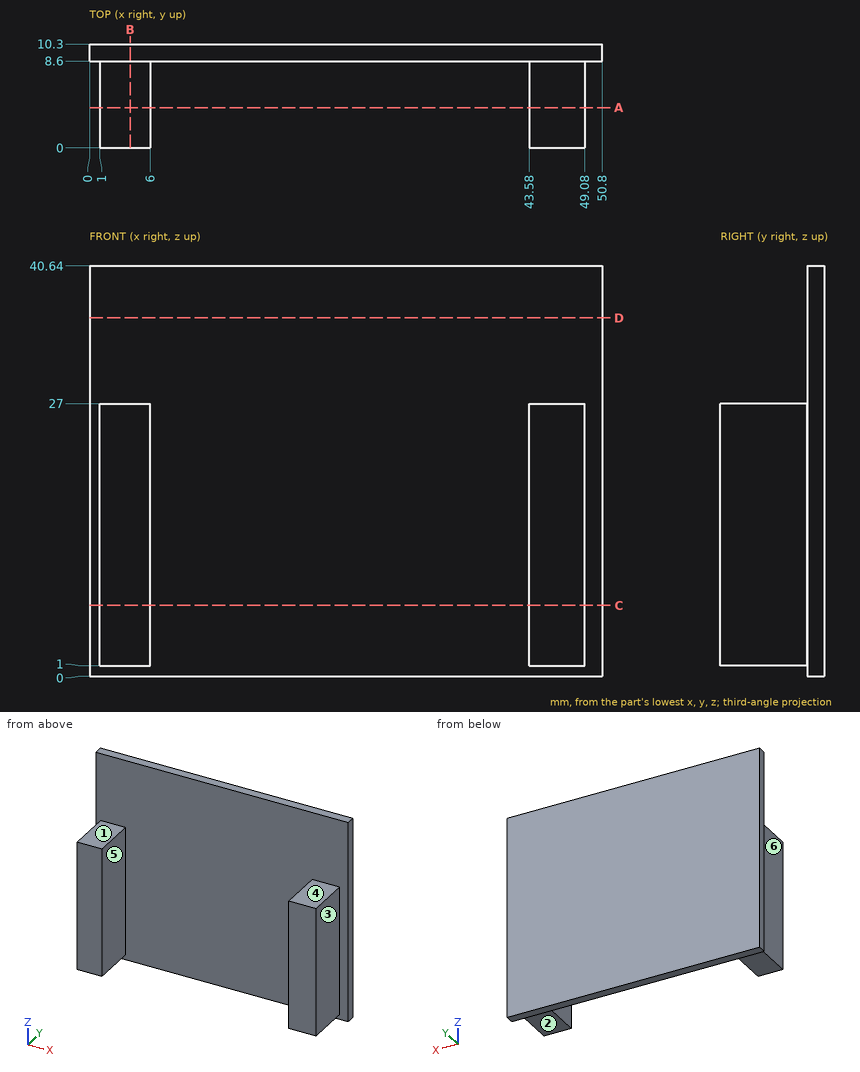
Design review of the part shown in the three views and the two pictorial views. Dimensions are in mm from the part's minimum x, y and z. A direction names the side the tool comes from. Give positions to 0.01 mm unless a question says otherwise; leave off trailing zeros. Order: outer loops, then holes, each group sorted by start corner. A loop starts at its lowest first (then second) coordinate and runs counter-clockwise, first axis right, second up. Notation, with made-up numbers: M -27,-34.75 L -5,-34.75 A28 cw -5,1.25 Z; hole C -36.5,9 d6. An arc over 180 degrees is marked long. Answer in a Markdown table with one row per item. Add a question column.
(1) Wall thickness on probe 1 along X at (y, z) = (8.25, 12); probe 2 along Y at (x, z) = (36.5, 32); probe 3 along Z at (x, y) = (47.5, 0.5): over which ranges is each line inside the solid? List them lowest first. Write a range as [from, to].
(2) For pin 1 (3 mm diameter, centred on y = 4.5, z = 21, fed in from +X); pin 2 (1 mm diameter, centred on x = 8, z = 23, fed in from -Y); pin 3 (1.6 mm diameter, centred on x = 45, y = 3.5, fed in from -Z), all flat-tipped, find the tip position at first contact; note any pin that passes through.
(3) Consider section D-D on z = 35.5. State the section outline as (x, y) points.
(4) Consider section A-A on y = 4. State the section outline as (x, z) points, and give its area (3 significant figures).
(5) For the marked faces 1, 2 and 3, list the 3-axis set-ups (+Z, -Z, +X, -X, +Y, -Y) from which the entire face can be reached by the end or side of a thin tool; tool diameter is ignored.
(6) Consider section C-C on z = 7. State the section outline as (x, y) points.
(7) Consider section B-B on x = 4. State the section outline as (y, z) points, and give its area (3 significant figures).
(8) Mouldability with a two-part tool opening along X and no side actions: class the marked faces 4, 5 and 6 as +X half, -X half, draft (parallel to the pull), parting line (faces both ways), or undercut.
Evaluation:
| question | item | result |
|---|---|---|
| 1 | probe 1 | x = [1, 6], [43.58, 49.08] |
| 1 | probe 2 | y = [8.6, 10.3] |
| 1 | probe 3 | z = [1, 27] |
| 2 | pin 1 | stops at x = 49.08 |
| 2 | pin 2 | stops at y = 8.6 |
| 2 | pin 3 | stops at z = 1 |
| 3 | outline | M 0,8.6 L 50.8,8.6 L 50.8,10.3 L 0,10.3 Z |
| 4 | outline | M 1,1 L 6,1 L 6,27 L 1,27 Z; M 43.58,1 L 49.08,1 L 49.08,27 L 43.58,27 Z |
| 4 | area | 273 mm^2 |
| 5 | face 1 | +Z, +X, -X, -Y |
| 5 | face 2 | -Z, +X, -X, -Y |
| 5 | face 3 | +Z, -Z, +X, -Y |
| 6 | outline | M 0,8.6 L 1,8.6 L 1,0 L 6,0 L 6,8.6 L 43.58,8.6 L 43.58,0 L 49.08,0 L 49.08,8.6 L 50.8,8.6 L 50.8,10.3 L 0,10.3 Z |
| 7 | outline | M 0,1 L 8.6,1 L 8.6,0 L 10.3,0 L 10.3,40.64 L 8.6,40.64 L 8.6,27 L 0,27 Z |
| 7 | area | 293 mm^2 |
| 8 | face 4 | draft |
| 8 | face 5 | undercut |
| 8 | face 6 | -X half |
